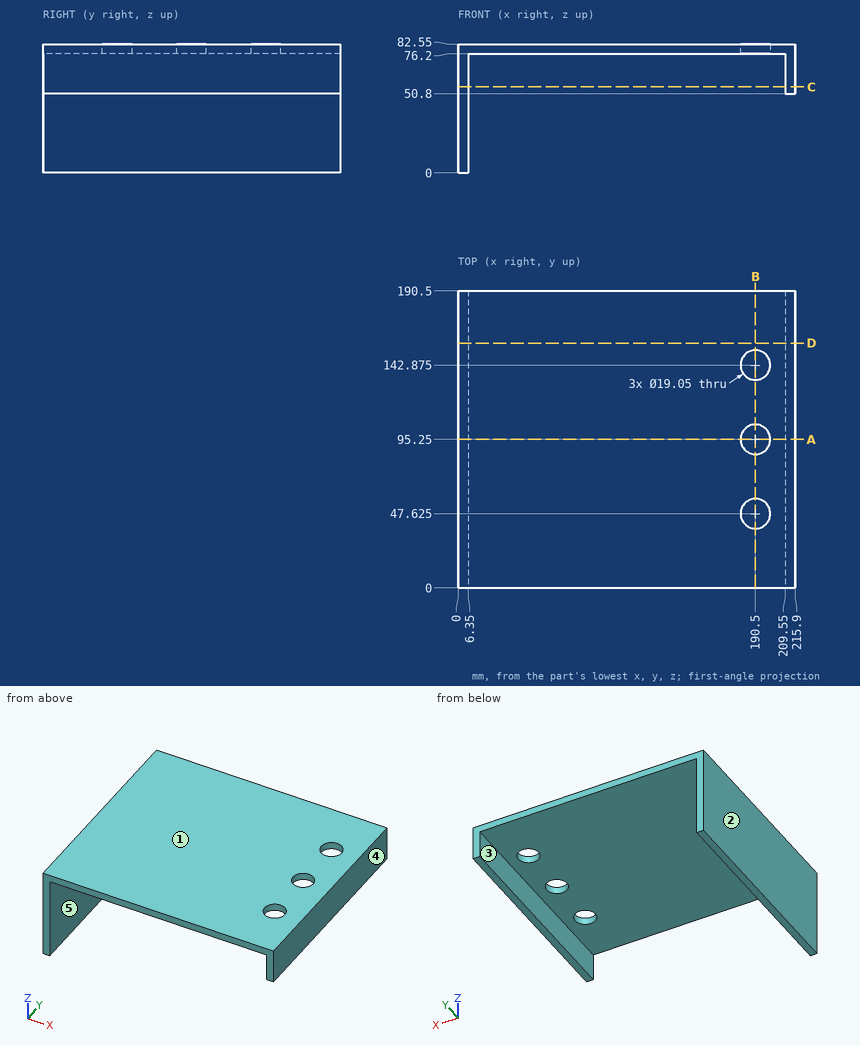
Check sheet for the drawn part. Datum: minimum x, y, z corner. Units: mm. A direction names the side the tool comes from. Coordinates: 2 decimals unless noted, no trailing zeros. Loops run counter-clockwise (first coordinate to the right, second up) from the corner with the lowest first, then second, coordinate; pieces in that order, holes last. Notation, with made-up numbers: (6.25, 76.25) -> (21.25, 76.25) arc R26 ccw to (21.25, 113.25) -> close; hole circle Ø7 at (84, 45). An arc over 180 degrees is marked (long way). Write each question's results on one line, items separated by ' | '.
Item 1: Section check D-D, the plane y = 157. Enter the section's corners in (x, z), plus the area to 3 significant figures.
Found:
outline: (0, 0) -> (6.35, 0) -> (6.35, 76.2) -> (209.55, 76.2) -> (209.55, 50.8) -> (215.9, 50.8) -> (215.9, 82.55) -> (0, 82.55) -> close | area: 2,020 mm2
Item 2: Gauge pin test, flat ends, axial feed: pin 1 (11.5 mm diameter, centred on x = 190.5, y = 142.875, fed in from -Z); pin 2 (8 mm diameter, centred on x = 30.5, y = 117, fed in from -Z); pin 3 (5 mm diameter, centred on x = 213.5, y = 97.5, fed in from -Z); pin 4 (5 mm diameter, centred on y = 101, z = 17.5, fed in from +X). Record the tip position at first contact, or that the pin passes through.
Found:
pin 1: passes through | pin 2: stops at z = 76.2 | pin 3: stops at z = 50.8 | pin 4: stops at x = 6.35
Item 3: Section check A-A, the plane y = 95.25. Enter the section's corners in (x, z) (3 decimals).
Found:
outline: (0, 0) -> (6.35, 0) -> (6.35, 76.2) -> (180.975, 76.2) -> (180.975, 82.55) -> (0, 82.55) -> close; (200.025, 76.2) -> (209.55, 76.2) -> (209.55, 50.8) -> (215.9, 50.8) -> (215.9, 82.55) -> (200.025, 82.55) -> close
Item 4: Tool access check on the marked faces 4 and 5. Record the directions out of +Z, -Z, +X, -X, +Y, -Y that give a thin tool (end or side, any length) a straight path to the whole face; none if there is none.
Found:
face 4: +Z, -Z, +X, +Y, -Y | face 5: -Z, +Y, -Y
Item 5: Section check C-C, the plane z = 55. Enter the section's corners in (x, y), plus the area to 3 significant figures.
Found:
outline: (0, 0) -> (6.35, 0) -> (6.35, 190.5) -> (0, 190.5) -> close; (209.55, 0) -> (215.9, 0) -> (215.9, 190.5) -> (209.55, 190.5) -> close | area: 2,420 mm2
Item 6: Mould release check, pull along X, two halves, no side actions. Record for the marked faces 1, 2 and 3: +X half, -X half, draft (parallel to the pull), parting line (faces both ways), or undercut.
Found:
face 1: draft | face 2: -X half | face 3: undercut
Item 7: Section check B-B, the plane x = 190.5. Enter the section's corners in (y, z) (3 decimals).
Found:
outline: (0, 76.2) -> (38.1, 76.2) -> (38.1, 82.55) -> (0, 82.55) -> close; (57.15, 76.2) -> (85.725, 76.2) -> (85.725, 82.55) -> (57.15, 82.55) -> close; (104.775, 76.2) -> (133.35, 76.2) -> (133.35, 82.55) -> (104.775, 82.55) -> close; (152.4, 76.2) -> (190.5, 76.2) -> (190.5, 82.55) -> (152.4, 82.55) -> close
Item 8: Material ranges on L1, parallel to Y at x = 190.5, z = 79.75 (3 decimals); L2, parallel to X at y = 176, z = 57; L3, parallel to Z at x = 182, y = 174, recorded low to high.
Found:
L1: y = 0 to 38.1, 57.15 to 85.725, 104.775 to 133.35, 152.4 to 190.5 | L2: x = 0 to 6.35, 209.55 to 215.9 | L3: z = 76.2 to 82.55
